Part model, mm, in its own coordinate system. Face numbers are marked on the shaded views. A direction names the side the tool comes from. Coordinates: 2 decimals unless noted, no trailing zeros. Loops run counter-clockwise (first coordinate to the right, second up) from the corner with the lowest first, then second, coordinate; pieces in that order, holes last. Notation, with made-up numbers: (79, -32.5) - (129, -32.5) arc R20 cw to (129, -21.5) - close; hole circle Ø10 at (54.5, 64). An arc over 180 degrees is marked (long way). Use a Markdown table: item, result. Add a question column.
1) Tool access for the marked faces 4, 5 and 6: list every direction of +Z, -Z, +X, -X, +Y, -Y with a clear straight run to the whole face (end or side of a thin tool).
2) Band-saw the part on A-A (z = 30.5). Give the cut face in (x, y).
3) Band-saw the part on B-B (x = 5). Give the cut face in (y, z), plus the area to 3 significant figures.
4) Probe probe 1 along Y at (x, z) = (2.75, 9.5); probe 2 along Y at (x, z) = (5.75, 27); probe 3 along X at (y, z) = (9.5, 10.5). List the from-to ranges inside material, lowest first. Write a range as [from, to].
5) Pull direction Y, two halves, no side cores. Call the marked faces 1, 2 and 3: +Y half, -Y half, draft (parallel to the pull), parting line (faces both ways), or undercut.
6) Band-saw the part on C-C (y = 9). Give the cut face in (x, z), plus the area to 4 significant figures.
7) Drop flat-ended pins along their axis: P1, Ø1.5, axis at y = 16, z = 32.5, coming from the +X side; P2, Ø3, axis at x = 6.5, z = 13.5, coming from the +Y side; P3, Ø4, axis at y = 13.5, z = 18.5, coming from the -X side. Give the stop position or say it passes through.
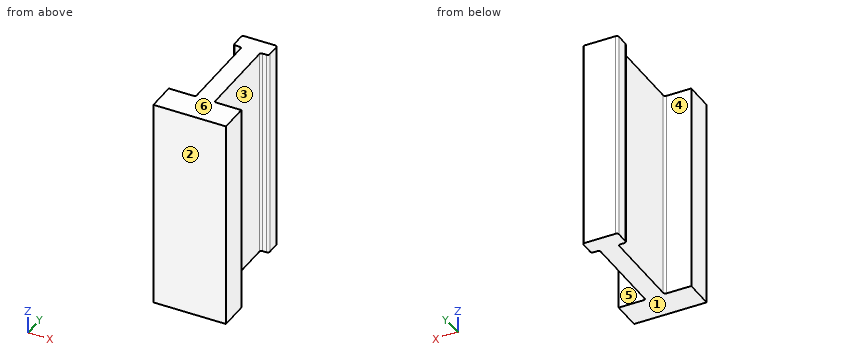
from build123d import *

# Parameters (mm, degrees)
BOSS_EXTRUDE1_DEPTH = 51


with BuildPart() as part:
    # Sketch1 → Boss-Extrude1 (new body)
    with BuildSketch(Plane.XY):
        with BuildLine():
            Line((8.75, -14), (-8.75, -14))
            Line((-8.75, -14), (-8.75, -7))
            Line((-8.75, -7), (-2.75, -7))
            ThreePointArc((-2.75, -7), (-2.396446609, -6.853553391), (-2.25, -6.5))
            Line((-2.25, -6.5), (-2.25, 13.5))
            ThreePointArc((-2.25, 13.5), (-2.396446609, 13.853553391), (-2.75, 14))
            Line((-2.75, 14), (-3.75, 14))
            ThreePointArc((-3.75, 14), (-4.103553391, 14.146446609), (-4.25, 14.5))
            Line((-4.25, 14.5), (-4.25, 17.5))
            ThreePointArc((-4.25, 17.5), (-4.103553391, 17.853553391), (-3.75, 18))
            Line((-3.75, 18), (3.75, 18))
            ThreePointArc((3.75, 18), (4.103553391, 17.853553391), (4.25, 17.5))
            Line((4.25, 17.5), (4.25, 14.5))
            ThreePointArc((4.25, 14.5), (4.103553391, 14.146446609), (3.75, 14))
            Line((3.75, 14), (2.75, 14))
            ThreePointArc((2.75, 14), (2.396446609, 13.853553391), (2.25, 13.5))
            Line((2.25, 13.5), (2.25, -6.5))
            ThreePointArc((2.25, -6.5), (2.396446609, -6.853553391), (2.75, -7))
            Line((2.75, -7), (8.75, -7))
            Line((8.75, -7), (8.75, -14))
        make_face()
    extrude(amount=BOSS_EXTRUDE1_DEPTH)


solid = part.part
Answer block:
| question | item | result |
|---|---|---|
| 1 | face 4 | +Z, -Z, -X |
| 1 | face 5 | +Z, -Z, +X |
| 1 | face 6 | +Z, +X, -X, +Y, -Y |
| 2 | outline | (-8.75, -14) - (8.75, -14) - (8.75, -7) - (2.75, -7) arc R0.5 cw to (2.25, -6.5) - (2.25, 13.5) arc R0.5 cw to (2.75, 14) - (3.75, 14) arc R0.5 ccw to (4.25, 14.5) - (4.25, 17.5) arc R0.5 ccw to (3.75, 18) - (-3.75, 18) arc R0.5 ccw to (-4.25, 17.5) - (-4.25, 14.5) arc R0.5 ccw to (-3.75, 14) - (-2.75, 14) arc R0.5 cw to (-2.25, 13.5) - (-2.25, -6.5) arc R0.5 cw to (-2.75, -7) - (-8.75, -7) - close |
| 3 | outline | (-14, 0) - (-7, 0) - (-7, 51) - (-14, 51) - close |
| 3 | area | 357 mm2 |
| 4 | probe 1 | [-14, -7], [14, 18] |
| 4 | probe 2 | [-14, -7] |
| 4 | probe 3 | [-2.25, 2.25] |
| 5 | face 1 | draft |
| 5 | face 2 | -Y half |
| 5 | face 3 | undercut |
| 6 | outline | (-2.25, 0) - (2.25, 0) - (2.25, 51) - (-2.25, 51) - close |
| 6 | area | 229.5 mm2 |
| 7 | P1 | x = 4.25 |
| 7 | P2 | y = -7 |
| 7 | P3 | x = -4.25 |
